```python
from build123d import *

# Parameters (mm, degrees)
SKETCH4_W         = 5.0419
SKETCH4_H         = 47.625
CIRPATTERN1_COUNT = 8


with BuildPart() as part:
    # Sketch1 → Revolve1 (revolve)
    with BuildSketch(Plane.XY, mode=Mode.PRIVATE) as revolve1_sk:
        with BuildLine():
            Line((0, 45.9613), (15.6972, 45.9613))
            Line((15.6972, 45.9613), (15.6972, 44.508928))
            Line((15.6972, 44.508928), (20.08759, 44.508928))
            ThreePointArc((20.08759, 44.508928), (20.518642294, 44.330380294), (20.69719, 43.899328))
            Line((20.69719, 43.899328), (20.69719, 41.783))
            Line((20.69719, 41.783), (22.8092, 41.783))
            Line((22.8092, 41.783), (22.8092, 38.1))
            Line((22.8092, 38.1), (55.88, 38.1))
            Line((55.88, 38.1), (55.88, 46.355))
            Line((55.88, 46.355), (54.61, 47.625))
            Line((54.61, 47.625), (31.75, 47.625))
            Line((31.75, 47.625), (31.75, 43.815))
            Line((31.75, 43.815), (24.5491, 43.815))
            Line((24.5491, 43.815), (24.5491, 47.625))
            Line((24.5491, 47.625), (0, 47.625))
            Line((0, 47.625), (0, 45.9613))
        make_face()
    revolve(revolve1_sk.sketch.rotate(Axis((0, 0, 0), (1, 0, 0)), 90), axis=Axis((0, 0, 0), (1, 0, 0)))

    # Sketch4 → Tap Drill for 3/8 Helicoil1 (revolve, cut)
    with BuildSketch(Plane.YZ.offset(43.18)):
        with Locations((2.52095, 23.8125)):
            Rectangle(SKETCH4_W, SKETCH4_H)
    tap_drill_for_3_8_helicoil1 = revolve(axis=Axis((43.18, 0, -6.35), (0, 0, 1)), mode=Mode.SUBTRACT)

    # CirPattern1: Tap Drill for 3/8 Helicoil1 ×8 about axis
    cirpattern1_axis = Axis((54.61, 0, 0), (-1, 0, 0))
    for i in range(1, CIRPATTERN1_COUNT):
        add(tap_drill_for_3_8_helicoil1.rotate(cirpattern1_axis, i * 360 / CIRPATTERN1_COUNT), mode=Mode.SUBTRACT)


solid = part.part
```
Here's how the part is built. I have some questions about the finished solid (model axes, mm). A direction names the side the tool comes from. Round coordinates to 2 decimals unless told otherwise and drop trailing zeros. Write each loop counter-clockwise with the first axis right and the second up, starting at its lowest first coordinate (ties: lowest second). Pieces come first, ordered by that corner, then holes.
Q1. Please list where these lines run through material, in increasing order: probe 1 along X at (y, z) = (0, -43); probe 2 along Y at (x, z) = (11, 0) (3 decimals); probe 3 along Y at (x, z) = (35, 0) (3 decimals).
Q2. If we section it at A-A on x = 43.18: Give the number of separate pieces and of enclosed holes in the cut face, plus the area to 3 significant figures.
Q3. If we mould it in two halves opening along Z, with no side actions, what happens to faces 3 (the flat face through (0, -39, -25)), 4 (the cylindrical face through (28.099, 42.773, -9.498)), 5 (the cylindrical face through (45.111, -33.532, -26.946))? For each: +Z half, -Z half, draft (parallel to the pull), parting line (faces both ways), or undercut.
Q4. If we section it at C-C on x = 33: Write out the boundary of the cut face in (y, z) (3 decimals), plus the area to 3 significant figures.
Q5. Will these pins go through, and if not, where does the flat tip stop? P1, Ø8, axis at x = 43.18, z = 0, coming from the -Y side; P2, Ø2, axis at x = 49, z = 33, coming from the -Y side; P3, Ø12, axis at x = 20, z = 24, coming from the +Y side; P4, Ø1, axis at x = 37, y = -14, coming from the -Z side.
Q6. Which directions (+Z, -Z, +X, -X, +Y, -Y) give clear straight access to the entire face, cutting with the end or side of a thin tool? Please do faces 1 (the flat face through (20.697, 16, 39)), 2 (the flat face through (55.88, 38, 7)).
Answer below:
1. probe 1: x = 20.7 to 38.14, 48.22 to 55.88
1. probe 2: y = -47.625 to -45.961, 45.961 to 47.625
1. probe 3: y = -47.625 to -38.1, 38.1 to 47.625
2. separate pieces: 8
2. enclosed holes: 0
2. area: 1,800 mm2
3. face 3: draft
3. face 4: parting line
3. face 5: undercut
4. outline: circle Ø95.25 at (0, 0); hole circle Ø76.2 at (0, 0)
4. area: 2,570 mm2
5. P1: passes through
5. P2: stops at y = -35.27
5. P3: stops at y = 44.09
5. P4: stops at z = -45.67
6. face 1: -X
6. face 2: +Z, -Z, +X, +Y, -Y
